Input: part model. Units: mm. Frame: model coordinates. A direction names the side the tool comes from. Coordinates: 2 decimals unless noted, no trailing zeros. Loops run counter-clockwise (first coordinate to the right, second up) from the corner with the lowest first, then second, coordinate; pieces in that order, holes last.
Item 1: Contact query for flat-ended pins moving along their axis: P1, Ø0.8, axis at y = 1.5, z = -1, coming from the +X side; P2, Ø0.5, axis at y = 2, z = -1, coming from the -X side; P3, Ø0.5, axis at x = -1, z = 1, coming from the +Y side; P4, Ø1.7, axis at x = 1.5, z = -1, coming from the +Y side. Output: stop coordinate, or through.
Item 2: Reachability of faces 1 (the flat face through (-0.4, 2, 1)), 2 (the flat face through (-1, 2, -0.4)), 3 (the flat face through (0.4, 2, 1)) from +Z, -Z, +X, -X, +Y, -Y: full face, straight path, thin tool, end or side. Return the list, or none.
Item 3: Section A-A on x = -0.8. Return loops of the section in (y, z), and give its area (3 significant figures).
Item 4: Section B-B on z = -1.55. Return loops of the section in (x, y).
Item 5: Ray query, line 1 along Y through (x, z) = (0.45, -0.8); line 2 along Z through (x, y) = (-1.7, 1). Return the intervals inside material, ascending.
```python
from build123d import *

# Parameters (mm, degrees)
SKETCH_5_W      = 0.8
SKETCH_5_H      = 3.9
SKETCH_5_W_2    = 3.9
SKETCH_5_H_2    = 0.8
EXTRUDE_1_DEPTH = 3.9
SKETCH_6_W      = 3.9
SKETCH_6_H      = 3.9
EXTRUDE_2_DEPTH = 10


with BuildPart() as part:
    # 草图5 → 凸台-拉伸1 (new body)
    with BuildSketch(Plane(origin=(0, 0, 0), x_dir=(-1, 0, 0), z_dir=(0, 1, 0))):
        Rectangle(SKETCH_5_W, SKETCH_5_H)
        Rectangle(SKETCH_5_W_2, SKETCH_5_H_2)
    extrude(amount=EXTRUDE_1_DEPTH)

    # 草图6 → 凸台-拉伸2 (add)
    with BuildSketch(Plane.XZ):
        Rectangle(SKETCH_6_W, SKETCH_6_H)
    extrude(amount=EXTRUDE_2_DEPTH)


solid = part.part
```
Results found:
1. P1: stops at x = 0.4
1. P2: stops at x = -0.4
1. P3: stops at y = 0
1. P4: stops at y = 3.9
2. face 1: +Z, -X, +Y
2. face 2: -Z, -X, +Y
2. face 3: +Z, +X, +Y
3. outline: (-10, -1.95) - (0, -1.95) - (0, -0.4) - (3.9, -0.4) - (3.9, 0.4) - (0, 0.4) - (0, 1.95) - (-10, 1.95) - close
3. area: 42.1 mm2
4. outline: (-1.95, -10) - (1.95, -10) - (1.95, 0) - (0.4, 0) - (0.4, 3.9) - (-0.4, 3.9) - (-0.4, 0) - (-1.95, 0) - close
5. line 1: y = -10 to 0
5. line 2: z = -0.4 to 0.4
